Here's how the part is built. I have some questions about the finished solid (model axes, mm). Face numbers are marked on the shaded views. A direction names the side the tool comes from. Round coordinates to 2 decimals unless told otherwise and drop trailing zeros. Write each loop counter-clockwise with the first axis right and the second up, starting at its lowest first coordinate (ties: lowest second). Pieces come first, ordered by that corner, then holes. Notation, with made-up numbers: (68.5, 44) -> (85.5, 44) arc R27 ccw to (85.5, 66) -> close; hole circle Ø6 at (26.25, -36.75). An arc over 180 degrees is marked (long way). Put each result on its own line as item: value. Start each with the question number.
1) Will these pins go through, and if not, where does the flat tip stop? P1, Ø4, axis at x = -3.5, y = 15.5, coming from the -Z side; P2, Ø12, axis at x = -10, z = 42, coming from the +Y side; P3, Ø17.5, axis at x = 0, y = -1, coming from the +Z side.
2) We'd pull the mould along Y, two halves only. Please class the marked faces 1, 2 and 3: released by +Y, released by -Y, zero draft, split by the parting line, or undercut.
3) Which directions (+Z, -Z, +X, -X, +Y, -Y) give clear straight access to the entire face, cutting with the end or side of a thin tool? Please do the marked faces 4, 5 and 6.
4) I want a section at B-B, the plane z = 13. List the corners of the cut face in (x, y) for me.
5) If I drill on line 1 along Z through (x, y) = (10, 15); line 2 along Z through (x, y) = (6.5, 8); line 3 along Z through (x, y) = (4, 10), over which ranges is the centre line in solid material (lowest first)? Write a range as [from, to].
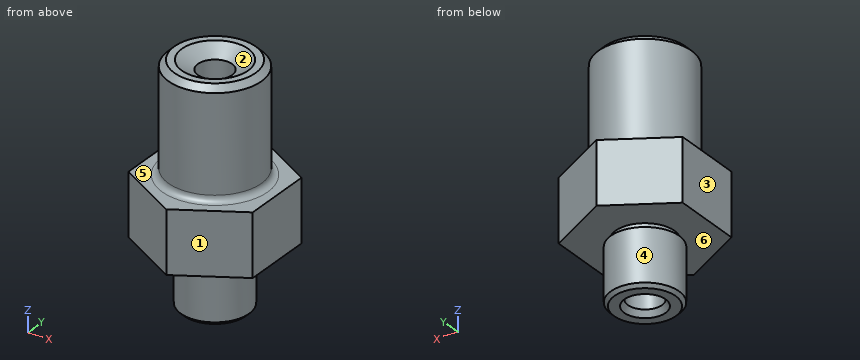
from build123d import *

# Parameters (mm, degrees)
SKETCH_1_R          = 17.5
EXTRUDE_1_DEPTH     = 20
SKETCH_2_R          = 15
EXTRUDE_2_DEPTH     = 35
SKETCH_3_R          = 11
EXTRUDE_3_DEPTH     = 20
CHAMFER_1_SIZE      = 1.1015
SKETCH_5_R          = 17.5
SKETCH_5_R_2        = 9.5
CUT_EXTRUDE_1_DEPTH = 2
CHAMFER_2_SIZE      = 1.921
FILLET_1_R          = 2
CHAMFER_3_SIZE      = 2
CHAMFER_3_SIZE2     = 1.154700538
SKETCH_6_R          = 17.5
EXTRUDE_4_DEPTH     = 20


with BuildPart() as part:
    # Эскиз1 → Бобышка-Вытянуть1 (new body)
    with BuildSketch(Plane.XY):
        Circle(SKETCH_1_R)
    extrude(amount=EXTRUDE_1_DEPTH)

    # Эскиз2 → Бобышка-Вытянуть2 (add)
    with BuildSketch(Plane.XY.offset(20)):
        Circle(SKETCH_2_R)
    extrude(amount=EXTRUDE_2_DEPTH)

    # Эскиз3 → Бобышка-Вытянуть3 (add)
    with BuildSketch(Plane(origin=(0, 0, 0), x_dir=(-1, 0, 0), z_dir=(0, 0, -1))):
        Circle(SKETCH_3_R)
    extrude(amount=EXTRUDE_3_DEPTH)

    # Эскиз4 → Вырез-Повернуть1 (revolve, cut)
    with BuildSketch(Plane(origin=(0, 0, 0), x_dir=(0, 0, -1), z_dir=(1, 0, 0))):
        Polygon((-55, 0), (-55, 10.696152423), (-52, 5.5), (20, 5.5), (20, 0), align=None)
    revolve(axis=Axis((0, 0, 55), (0, 0, -1)), mode=Mode.SUBTRACT)

    # Фаска1
    chamfer_1_edges = [part.edges().sort_by_distance(p)[0] for p in [
        (11, 0, -20),
    ]]
    chamfer(chamfer_1_edges, length=CHAMFER_1_SIZE)

    # Эскиз5 → Вырез-Вытянуть1 (cut)
    with BuildSketch(Plane(origin=(0, 0, 0), x_dir=(-1, 0, 0), z_dir=(0, 0, -1))):
        Circle(SKETCH_5_R)
        Circle(SKETCH_5_R_2, mode=Mode.SUBTRACT)
    extrude(amount=CUT_EXTRUDE_1_DEPTH, mode=Mode.SUBTRACT)

    # Фаска2
    chamfer_2_edges = [part.edges().sort_by_distance(p)[0] for p in [
        (-15, 0, 55),
    ]]
    chamfer(chamfer_2_edges, length=CHAMFER_2_SIZE)

    # Скругление1
    fillet_1_edges = [part.edges().sort_by_distance(p)[0] for p in [
        (-15, 0, 20),
    ]]
    fillet(fillet_1_edges, radius=FILLET_1_R)

    # Фаска3
    chamfer_3_edges = [part.edges().sort_by_distance(p)[0] for p in [
        (0, -5.5, -20),
    ]]
    chamfer_3_side = [part.faces().sort_by_distance(p)[0] for p in [
        (0, -5.5, 16),
    ]]
    chamfer(chamfer_3_edges, length=CHAMFER_3_SIZE, length2=CHAMFER_3_SIZE2, reference=chamfer_3_side[0])

    # Эскиз6 → Бобышка-Вытянуть4 (add)
    with BuildSketch(Plane(origin=(0, 0, 0), x_dir=(-1, 0, 0), z_dir=(0, 0, -1))):
        Polygon((0, 23.094010768), (-20, 11.547005384), (-20, -11.547005384), (0, -23.094010768), (20, -11.547005384), (20, 11.547005384), align=None)
        Circle(SKETCH_6_R, mode=Mode.SUBTRACT)
    extrude(amount=-EXTRUDE_4_DEPTH)


solid = part.part
Findings:
1. P1: stops at z = 0
1. P2: stops at y = 14.46
1. P3: stops at z = 54.45
2. face 1: released by -Y
2. face 2: undercut
2. face 3: zero draft
3. face 4: -Z
3. face 5: +Z
3. face 6: none
4. outline: (-20, -11.55) -> (0, -23.09) -> (20, -11.55) -> (20, 11.55) -> (0, 23.09) -> (-20, 11.55) -> close; hole circle Ø11 at (0, 0)
5. line 1: z = [0, 20]
5. line 2: z = [-19.59, -2], [0, 54.78]
5. line 3: z = [-19.13, -2], [0, 55]
